Part model, mm, in its own coordinate system. Coordinates: 2 decimals unless noted, no trailing zeros. Write each loop counter-clockwise with the first axis right and the second up, starting at its lowest first coordinate (ties: lowest second). Pieces come first, ordered by that corner, then holes. Notation, with made-up numbers: (44, -36.75) - (73, -36.75) arc R11 ccw to (73, -24.75) - close; hole circle Ø4 at (-11.5, 10.5). An arc over 180 degrees is marked (long way). Use a Markdown table: item, result.
```python
from build123d import *

# Parameters (mm, degrees)
F1_R     = 10
F3_DEPTH = 10
F2_R     = 10
F4_DEPTH = 10
F5_DEPTH = 10
F6_W     = 16
F6_H     = 16
F7_DEPTH = 10


with BuildPart() as f3:
    # F1 (on Top) → F3 (new body, symmetric)
    with BuildSketch(Plane.XY):
        Circle(F1_R)
    extrude(amount=F3_DEPTH, both=True)

    # F2 (on Right) → F4 (intersect, symmetric)
    with BuildSketch(Plane.YZ):
        Circle(F2_R)
    extrude(amount=F4_DEPTH, both=True, mode=Mode.INTERSECT)

    # F0 (on Front) → F5 (intersect, symmetric)
    with BuildSketch(Plane.XZ):
        with BuildLine():
            ThreePointArc((0, -10), (7.071068, -7.071068), (10, 0))
            ThreePointArc((10, 0), (7.071068, 7.071068), (0, 10))
            ThreePointArc((0, 10), (-7.071068, 7.071068), (-10, 0))
            ThreePointArc((-10, 0), (-7.071068, -7.071068), (0, -10))
        make_face()
    extrude(amount=F5_DEPTH, both=True, mode=Mode.INTERSECT)

    # F6 (on Top) → F7 (intersect, symmetric)
    with BuildSketch(Plane.XY):
        Rectangle(F6_W, F6_H)
    extrude(amount=F7_DEPTH, both=True, mode=Mode.INTERSECT)


solid = f3.part
```
Item 1: Band-saw the part on A-A, the plane z = -5.5. Give the cut face in (x, y), then the cut area to 3 significant figures.
From the geometry:
| item | result |
|---|---|
| outline | (-8, -6) arc R10 ccw to (-6, -8) - (6, -8) arc R10 ccw to (8, -6) - (8, 6) arc R10 ccw to (6, 8) - (-6, 8) arc R10 ccw to (-8, 6) - close |
| area | 249 mm^2 |
Item 2: Band-saw the part on D-D, the plane z = 7.75. Give the cut face in (x, y), then the cut area to 3 significant figures.
From the geometry:
| item | result |
|---|---|
| outline | (-6.32, -6.32) - (6.32, -6.32) - (6.32, 6.32) - (-6.32, 6.32) - close |
| area | 160 mm^2 |
Item 3: Band-saw the part on C-C, the plane z = -8. Give the cut face in (x, y), then the cut area to 3 significant figures.
From the geometry:
| item | result |
|---|---|
| outline | (-6, -6) - (6, -6) - (6, 6) - (-6, 6) - close |
| area | 144 mm^2 |
Item 4: Drill centre lines: probe 1 along Y at (x, z) = (4, -8); probe 2 along Z at (x, y) = (1.5, 3.25); probe 3 along Z at (x, y) = (-7.25, 5.25). Where is each one in solid material? Low to high.
From the geometry:
| item | result |
|---|---|
| probe 1 | -6 to 6 |
| probe 2 | -9.46 to 9.46 |
| probe 3 | -6.89 to 6.89 |
Item 5: Band-saw the part on B-B, the plane y = -6.25. Give the cut face in (x, z).
From the geometry:
| item | result |
|---|---|
| outline | (-7.81, -6.25) arc R10 ccw to (-6.25, -7.81) - (6.25, -7.81) arc R10 ccw to (7.81, -6.25) - (7.81, 6.25) arc R10 ccw to (6.25, 7.81) - (-6.25, 7.81) arc R10 ccw to (-7.81, 6.25) - close |
Item 6: Drop a flat-ended pin along its axis: P1, Ø1.5, axis at x = 5.5, y = 3.5, coming from the -Z side. Give the stop position or say it passes through.
From the geometry:
| item | result |
|---|---|
| P1 | z = -8.8 |
